```python
from build123d import *

# Parameters (mm, degrees)
BOSS_EXTRUDE1_DEPTH = 11.1125
SKETCH2_R           = 5.55625
CUT_EXTRUDE1_DEPTH  = 54.549874163


with BuildPart() as part:
    # Sketch1 → Boss-Extrude1 (new, symmetric)
    with BuildSketch(Plane.XY):
        with BuildLine():
            Line((-12.22375, 50.06975), (12.22375, 50.06975))
            ThreePointArc((12.22375, 50.06975), (14.550144612, 49.055424226), (15.390100159, 46.660545659))
            Line((15.390100159, 46.660545659), (11.873813095, -0.878266277))
            ThreePointArc((11.873813095, -0.878266277), (0.015148097, -11.906240364), (-11.871539853, -0.908477065))
            Line((-11.871539853, -0.908477065), (-15.389493961, 45.062449449))
            ThreePointArc((-15.389493961, 45.062449449), (-14.552891714, 47.462422649), (-12.22375, 48.47971))
            Line((-12.22375, 48.47971), (12.22375, 48.47971))
            Line((12.22375, 48.47971), (12.22375, 46.89221))
            Line((12.22375, 46.89221), (-12.22375, 46.89221))
            ThreePointArc((-12.22375, 46.89221), (-13.388320857, 46.383566325), (-13.80662198, 45.183579725))
            Line((-13.80662198, 45.183579725), (-10.288667873, -0.78734679))
            ThreePointArc((-10.288667873, -0.78734679), (0.01312835, -10.318741649), (10.290638015, -0.761164107))
            Line((10.290638015, -0.761164107), (13.806925079, 46.77764783))
            ThreePointArc((13.806925079, 46.77764783), (13.386947306, 47.975087113), (12.22375, 48.48225))
            Line((12.22375, 48.48225), (-12.22375, 48.48225))
            Line((-12.22375, 48.48225), (-12.22375, 50.06975))
        make_face()
    extrude(amount=BOSS_EXTRUDE1_DEPTH, both=True)

    # Sketch2 → Cut-Extrude1 (cut, through all)
    with BuildSketch(Plane(origin=(0, 0, 0), x_dir=(1, 0, 0), z_dir=(0, 1, 0))):
        with Locations(Location((0, 0, 0), (0, 0, 180))):
            Circle(SKETCH2_R)
    extrude(amount=CUT_EXTRUDE1_DEPTH, mode=Mode.SUBTRACT)


solid = part.part
```
Design review of the part built by this model. Coordinates are the model's own, in mm. A direction names the side the tool comes from. Coordinates: 2 decimals unless noted, no trailing zeros. Order: outer loops, then holes, each group sorted by start corner. A loop starts at its lowest first (then second) coordinate and runs counter-clockwise, first axis right, second up.
1) Take a section at A-A, the plane x = 13. Give the boundary of the cut face in (y, z), and give its area (3 significant figures).
2) Clearance check with flat-ended pins moving along their axes: pin 1 (5 mm diameter, centred on x = 4, z = 1, fed in from -Y); pin 2 (6.5 mm diameter, centred on x = 4, z = 1, fed in from -Y); pin 3 (0.5 mm diameter, centred on y = 49.5, z = -5, fed in from -X). State where each tip first meets the part, or that it passes through.
3) Take a section at B-B, the plane y = 4. Give the boundary of the cut face in (x, z), and give its area (3 significant figures).
4) Wall thickness on line 1 along Z through (x, y) = (0, 49.3); line 2 along X through (y, z) = (47.65, 0); line 3 along X through (y, z) = (47.8, 0): over which ranges is each line inside the solid? List them lowest first.
5) Mouldability with a two-part tool opening along Y and no side actions: class faces 5 (the cylindrical face through (0.264, -11.903, 0.156)), 6 (the flat face through (-6, 50.07, 0)), 7 (the flat face through (6, 46.892, 0)) as +Y half, -Y half, draft (parallel to the pull), parting line (faces both ways), or undercut.
6) Take a section at C-C, the plane z = 1.25. State how many separate pieces and enclosed holes the cut face has, and give its area (3 significant figures).
7) For faces 1 (the flat face through (13, 22, 11.112)), 2 (the flat face through (12.224, 48, 0)), 3 (the flat face through (-12.224, 49, 0)), 4 (the cylindrical face through (4.095, 49.265, 3.755)), list the 3-axis set-ups (+Z, -Z, +X, -X, +Y, -Y) from which the entire face can be reached by the end or side of a thin tool; tool diameter is ignored.
8) Take a section at D-D, the plane x = 0. Give the boundary of the cut face in (y, z), and give its area (3 significant figures).
Returned:
1. outline: (14.35, -11.11) - (35.87, -11.11) - (35.87, 11.11) - (14.35, 11.11) - close; (48.28, -11.11) - (49.97, -11.11) - (49.97, 11.11) - (48.28, 11.11) - close
1. area: 516 mm2
2. pin 1: stops at y = -11.81
2. pin 2: stops at y = -11.88
2. pin 3: stops at x = -12.22
3. outline: (-12.25, -11.11) - (-10.66, -11.11) - (-10.66, 11.11) - (-12.25, 11.11) - close; (10.64, -11.11) - (12.23, -11.11) - (12.23, 11.11) - (10.64, 11.11) - close
3. area: 70.8 mm2
4. line 1: z = -11.11 to -5.56, 5.56 to 11.11
4. line 2: x = -14.36 to -5.56, 5.56 to 12.22, 13.62 to 15.31
4. line 3: x = -14.19 to -5.56, 5.56 to 12.22, 13.53 to 15.27
5. face 5: -Y half
5. face 6: +Y half
5. face 7: undercut
6. separate pieces: 3
6. enclosed holes: 0
6. area: 257 mm2
7. face 1: +Z, +X, -X, +Y, -Y
7. face 2: +Z, -Z
7. face 3: +Z, -Z, -X, +Y
7. face 4: +Y
8. outline: (-11.91, -11.11) - (-10.32, -11.11) - (-10.32, 11.11) - (-11.91, 11.11) - close; (46.89, -11.11) - (48.48, -11.11) - (48.48, -5.56) - (46.89, -5.56) - close; (46.89, 5.56) - (48.48, 5.56) - (48.48, 11.11) - (46.89, 11.11) - close; (48.48, -11.11) - (50.07, -11.11) - (50.07, -5.56) - (48.48, -5.56) - close; (48.48, 5.56) - (50.07, 5.56) - (50.07, 11.11) - (48.48, 11.11) - close
8. area: 70.6 mm2
